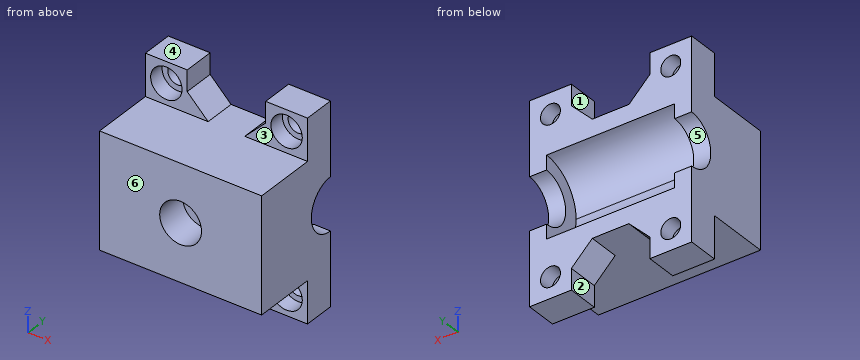
```python
from build123d import *

# Parameters (mm, degrees)
SKETCH1_W                 = 31
SKETCH1_H                 = 22
BOSS_EXTRUDE1_DEPTH       = 11
SKETCH2_W                 = 31
SKETCH2_H                 = 22
SKETCH2_R                 = 4
BOSS_EXTRUDE2_DEPTH       = 7
SKETCH3_W                 = 24.5
SKETCH3_H                 = 15.5
CUT_EXTRUDE1_DEPTH        = 7.75
FILLET1_R                 = 7.75
CUT_EXTRUDE2_DEPTH        = 32.812929761
CUT_EXTRUDE2_DEPTH_BACK   = 32.812929761
SKETCH4_R                 = 5
SKETCH5_W                 = 8
SKETCH5_H                 = 8
SKETCH5_R                 = 1.905800151
BOSS_EXTRUDE3_DEPTH       = 6
CUT_EXTRUDE3_START        = -3
SKETCH6_R                 = 3
SKETCH6_R_2               = 1.905800151
CUT_EXTRUDE3_DEPTH        = 3
MIRROR9_COPY_1_SKETCH_W   = 8
MIRROR9_COPY_1_SKETCH_H   = 8
MIRROR9_COPY_1_SKETCH_R   = 1.905800151
MIRROR9_COPY_1_DEPTH      = 6
MIRROR9_START             = -3
MIRROR9_COPY_2_SKETCH_R   = 3
MIRROR9_COPY_2_SKETCH_R_2 = 1.905800151
MIRROR9_COPY_2_DEPTH      = 3
CHAMFER2_SIZE             = 4
SKETCH7_R                 = 4
BOSS_EXTRUDE4_DEPTH       = 1


with BuildPart() as part:
    # Sketch1 → Boss-Extrude1 (new body)
    with BuildSketch(Plane(origin=(0, 0, 0), x_dir=(1, 0, 0), z_dir=(0, 1, 0))):
        Rectangle(SKETCH1_W, SKETCH1_H)
    extrude(amount=BOSS_EXTRUDE1_DEPTH)

    # Sketch2 → Boss-Extrude2 (add)
    with BuildSketch(Plane(origin=(0, 0, 0), x_dir=(1, 0, 0), z_dir=(0, 1, 0))):
        Rectangle(SKETCH2_W, SKETCH2_H)
        with Locations(Location((0, 0, 0), (0, 0, 270))):
            Circle(SKETCH2_R, mode=Mode.SUBTRACT)
    extrude(amount=-BOSS_EXTRUDE2_DEPTH)

    # Sketch3 → Cut-Extrude1 (cut)
    with BuildSketch(Plane(origin=(0, 11, 0), x_dir=(1, 0, 0), z_dir=(0, 1, 0))):
        Rectangle(SKETCH3_W, SKETCH3_H)
    extrude(amount=-CUT_EXTRUDE1_DEPTH, mode=Mode.SUBTRACT)

    # Fillet1
    fillet1_edges = [part.edges().sort_by_distance(p)[0] for p in [
        (0, 3.25, 7.75),
        (0, 3.25, -7.75),
    ]]
    fillet(fillet1_edges, radius=FILLET1_R - 0.0001)  # a hair under: the kernel refuses the full size

    # Sketch4 → Cut-Extrude2 (cut, two sides: drawn at the far end of the back side and taken through both)
    with BuildSketch(Plane(origin=(-12.25, 0, 0), x_dir=(0, 0, -1), z_dir=(1, 0, 0)).offset(-CUT_EXTRUDE2_DEPTH_BACK)):
        with Locations((0, 11)):
            Circle(SKETCH4_R)
    extrude(amount=CUT_EXTRUDE2_DEPTH + CUT_EXTRUDE2_DEPTH_BACK, mode=Mode.SUBTRACT)

    # Sketch5 → Boss-Extrude3 (add)
    with BuildSketch(Plane(origin=(0, 11, 0), x_dir=(1, 0, 0), z_dir=(0, 1, 0))):
        with Locations((11.5, -15)):
            Rectangle(SKETCH5_W, SKETCH5_H)
        with Locations(Location((11.5, -15, 0), (0, 0, 270))):
            Circle(SKETCH5_R, mode=Mode.SUBTRACT)
    boss_extrude3 = extrude(amount=-BOSS_EXTRUDE3_DEPTH)

    # Sketch6 → Cut-Extrude3 (cut)
    with BuildSketch(Plane.XZ.offset(-5).offset(CUT_EXTRUDE3_START)):
        with Locations(Location((11.5, 15, 0), (0, 0, 270))):
            Circle(SKETCH6_R)
        with Locations(Location((11.5, 15, 0), (0, 0, 90))):
            Circle(SKETCH6_R_2, mode=Mode.SUBTRACT)
    cut_extrude3 = extrude(amount=CUT_EXTRUDE3_DEPTH, mode=Mode.SUBTRACT)

    # Mirror8: Boss-Extrude3, Cut-Extrude3 across plane
    add(boss_extrude3.mirror(Plane(origin=(0, 0, 0), x_dir=(0, 0, 1), z_dir=(1, 0, 0))))
    add(cut_extrude3.mirror(Plane(origin=(0, 0, 0), x_dir=(0, 0, 1), z_dir=(1, 0, 0))), mode=Mode.SUBTRACT)

    # Mirror9: Boss-Extrude3, Cut-Extrude3 across plane
    add(boss_extrude3.mirror(Plane.XY))
    add(cut_extrude3.mirror(Plane.XY), mode=Mode.SUBTRACT)

    # Mirror9 copy 1 sketch → Mirror9 copy 1 (add)
    with BuildSketch(Plane(origin=(0, 11, 0), x_dir=(-1, 0, 0), z_dir=(0, 1, 0))):
        with Locations((11.5, -15)):
            Rectangle(MIRROR9_COPY_1_SKETCH_W, MIRROR9_COPY_1_SKETCH_H)
        with Locations(Location((11.5, -15, 0), (0, 0, 270))):
            Circle(MIRROR9_COPY_1_SKETCH_R, mode=Mode.SUBTRACT)
    extrude(amount=-MIRROR9_COPY_1_DEPTH)

    # Mirror9 copy 2 sketch → Mirror9 copy 2 (cut)
    with BuildSketch(Plane(origin=(0, 5, 0), x_dir=(-1, 0, 0), z_dir=(0, -1, 0)).offset(MIRROR9_START)):
        with Locations(Location((11.5, 15, 0), (0, 0, 270))):
            Circle(MIRROR9_COPY_2_SKETCH_R)
        with Locations(Location((11.5, 15, 0), (0, 0, 90))):
            Circle(MIRROR9_COPY_2_SKETCH_R_2, mode=Mode.SUBTRACT)
    extrude(amount=MIRROR9_COPY_2_DEPTH, mode=Mode.SUBTRACT)

    # Chamfer2
    chamfer2_edges = [part.edges().sort_by_distance(p)[0] for p in [
        (-7.5, 8, -11),
        (7.5, 8, -11),
        (7.5, 8, 11),
        (-7.5, 8, 11),
    ]]
    chamfer(chamfer2_edges, length=CHAMFER2_SIZE)

    # Sketch7 → Boss-Extrude4 (add)
    with BuildSketch(Plane.XZ):
        with Locations(Location((0, 0, 0), (0, 0, 90))):
            Circle(SKETCH7_R)
    extrude(amount=BOSS_EXTRUDE4_DEPTH)


solid = part.part
```
Geometry check sheet. Reference: the model listing, model coordinates, mm. Face numbers are marked on the shaded views. A direction names the side the tool comes from. Give positions to 0.01 mm unless a question says otherwise; leave off trailing zeros. Write each loop counter-clockwise with the first axis right and the second up, starting at its lowest first coordinate (ties: lowest second). Pieces come first, ordered by that corner, then holes.
1) Section check C-C, the plane y = -4. Record the boundary of the cut face in (x, z).
2) Material ranges on L1, parallel to X at y = 9.45, z = 15; L2, parallel to Z at x = 0, y = -4.4; L3, parallel to Z at x = 11.5, y = 9.05, recorded low to high.
3) Section check A-A, the plane y = 8.75. State how many separate pieces and enclosed holes the cut face has, and give its area (3 significant figures).
4) Section check D-D, the plane z = 14. Record the boundary of the cut face in (x, y).
5) Access from +Z, -Z, +X, -X, +Y, -Y to the whole of each face (thin tool, end or side, straight path). Record for the marked faces 1, 2 and 3.
6) Release check for a two-part mould opening along Z. For the marked faces 4, 5 and 6 record: pulls with the +Z half, pulls with the -Z half, needs draft (parallel to the pull), parting line crosses it, or undercut.
7) Gauge pin test, flat ends, axial feed: pin 1 (5.5 mm diameter, centred on x = 0.5, y = 5.5, fed in from -Z); pin 2 (1.8 mm diameter, centred on x = -12.5, z = 15.5, fed in from -Y); pin 3 (7 mm diameter, centred on x = 11.5, z = 15, fed in from -Y). Record the tip position at first contact, or that the pin passes through.
Computed:
1. outline: (-15.5, -11) - (15.5, -11) - (15.5, 11) - (-15.5, 11) - close; hole circle Ø8 at (0, 0)
2. L1: x = -15.5 to -13.41, -9.59 to -7.5, 7.5 to 9.59, 13.41 to 15.5
2. L2: z = -11 to -4, 4 to 11
2. L3: z = -19 to -16.91, -13.09 to -7.5, 7.5 to 13.09, 16.91 to 19
3. separate pieces: 2
3. enclosed holes: 4
3. area: 503 mm2
4. outline: (-15.5, 5) - (-14.33, 5) - (-14.33, 8) - (-13.12, 8) - (-13.12, 11) - (-15.5, 11) - close; (-9.88, 8) - (-8.67, 8) - (-8.67, 5) - (-6.5, 5) - (-6.5, 11) - (-9.88, 11) - close; (6.5, 5) - (8.67, 5) - (8.67, 8) - (9.88, 8) - (9.88, 11) - (6.5, 11) - close; (13.12, 8) - (14.33, 8) - (14.33, 5) - (15.5, 5) - (15.5, 11) - (13.12, 11) - close
5. face 1: +Z, +Y, -Y
5. face 2: -Z, +Y, -Y
5. face 3: +Z, +X, -X, -Y
6. face 4: pulls with the +Z half
6. face 5: undercut
6. face 6: needs draft
7. pin 1: stops at z = -11
7. pin 2: stops at y = 8
7. pin 3: stops at y = 5
